```python
from build123d import *

# Parameters (mm, degrees)
F0_W      = 25
F0_H      = 60
F1_DEPTH  = 20
F2_W      = 10
F2_H      = 18
F3_DEPTH  = 25.001
F4_W      = 5
F4_H      = 7
F5_DEPTH  = 25.001
F7_D      = 3.1
F9_D      = 9.5
F9_DEPTH  = 35
F9_TIP    = 2.8540879404
F11_DEPTH = 20.001
F13_D     = 5
F13_DEPTH = 15
F13_TIP   = 1.5021515476
F14_DEPTH = 3
F15_W     = 10
F15_H     = 11
F16_DEPTH = 5.001


with BuildPart() as f1:
    # F0 (on Front) → F1 (new body)
    with BuildSketch(Plane.XZ):
        with Locations((12.5, -30)):
            Rectangle(F0_W, F0_H)
    extrude(amount=F1_DEPTH)

    # F2 (on face) → F3 (cut, through all)
    with BuildSketch(Plane(origin=(0, 0, 0), x_dir=(0, -1, 0), z_dir=(-1, 0, 0))):
        with Locations((10, -9)):
            Rectangle(F2_W, F2_H)
    extrude(amount=-F3_DEPTH, mode=Mode.SUBTRACT)

    # F4 (on face) → F5 (cut, through all)
    with BuildSketch(Plane(origin=(0, 0, 0), x_dir=(0, -1, 0), z_dir=(-1, 0, 0))):
        with Locations((2.5, -3.5)):
            Rectangle(F4_W, F4_H)
    extrude(amount=-F5_DEPTH, mode=Mode.SUBTRACT)

    # F7 (through all)
    with Locations(Plane(origin=(0, 0, 0), x_dir=(-1, 0, 0), z_dir=(0, 1, 0))):
        with Locations((-17.5, -11)):
            Hole(F7_D / 2)

    # F9
    with Locations(Plane.XY.offset(-18)):
        with Locations((5.5, -10)):
            Hole(F9_D / 2, depth=F9_DEPTH)
            with Locations((0, 0, -(F9_DEPTH + F9_TIP / 2))):  # 118° drill point
                Cone(0, F9_D / 2, F9_TIP, mode=Mode.SUBTRACT)

    # F10 (on face) → F11 (cut, through all)
    with BuildSketch(Plane.XZ.offset(20)):
        with BuildLine():
            Line((17.5, -1), (15, -1))
            ThreePointArc((15, -1), (13, -3), (15, -5))
            Line((15, -5), (17.5, -5))
            ThreePointArc((17.5, -5), (19.5, -3), (17.5, -1))
        make_face()
    extrude(amount=-F11_DEPTH, mode=Mode.SUBTRACT)

    # F13
    with Locations(Plane(origin=(0, 0, 0), x_dir=(-1, 0, 0), z_dir=(0, 1, 0))):
        with Locations((-17.5, -54), (-17.5, -22)):
            Hole(F13_D / 2, depth=F13_DEPTH)
            with Locations((0, 0, -(F13_DEPTH + F13_TIP / 2))):  # 118° drill point
                Cone(0, F13_D / 2, F13_TIP, mode=Mode.SUBTRACT)

    # F14 (add): a face of the model
    f14_faces = [f1.faces().sort_by_distance(p)[0] for p in [
        (12.5, -17.5, 0),
    ]]
    extrude(f14_faces, amount=F14_DEPTH)

    # F15 (on face) → F16 (cut, through all)
    with BuildSketch(Plane.XZ.offset(5)):
        with Locations((5, -12.5)):
            Rectangle(F15_W, F15_H)
    extrude(amount=-F16_DEPTH, mode=Mode.SUBTRACT)


solid = f1.part
```
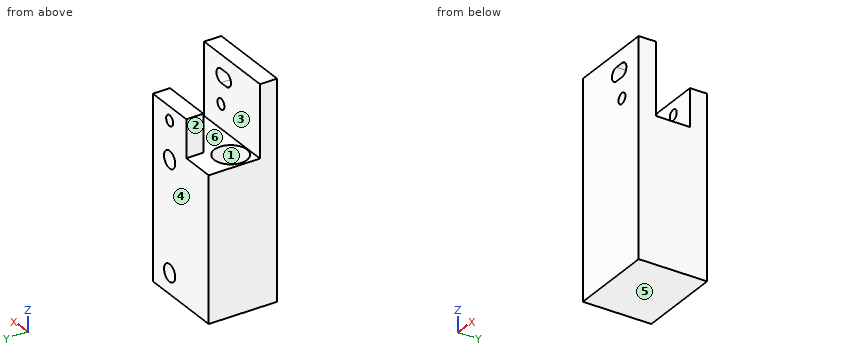
Could you check a few things on this model? Use its own coordinates, in mm. Face numbers are marked on the shaded views. A direction names the side the tool comes from. Round coordinates to 2 decimals unless told otherwise and drop trailing zeros. Order: outer loops, then holes, each group sorted by start corner. A loop starts at its lowest first (then second) coordinate and runs counter-clockwise, first axis right, second up. Notation, with made-up numbers: M 74,58 L 121,58 A24 cw 121,97 Z; hole C 40.25,65 d2. An arc over 180 degrees is marked long. One line per question, with ' | ' between items. Start each with the question number.
(1) Thinking about a two-plate mould opening in Y: for the marked faces 4, 5 and 6, which applies, +Y half, -Y half, draft (parallel to the pull), parting line (faces both ways), or undercut?
(2) Suppose I cut it at B-B on z = -37.5. List the corners of the cut face in (x, y) for me.
(3) Suppose I cut it at C-C on x = 12. List the corners of the cut face in (y, z) for me, then the cut area to 3 significant figures.
(4) Suppose I cut it at A-A on y = -4.25. List the corners of the cut face in (x, z) for me.
(5) For the marked faces 1, 2 and 3, which set-ups out of +Z, -Z, +X, -X, +Y, -Y let a thin tool reach every point of the face, with its end or its side?
(6) Suppose I cut it at D-D on z = -6. List the corners of the cut face in (x, y) for me.
(7) Please list where these lines run through material, in increasing order: line 1 along Z through (x, y) = (17.5, -9.25); line 2 along Z through (x, y) = (17.5, -17); line 3 along Z through (x, y) = (17.5, -1.45).
(8) For P1, Ø2.5, axis at y = -2.5, z = -14, coming from the -X side; P2, Ø3, axis at x = 17.5, z = -54, coming from the +Y side; P3, Ø10, axis at x = 13.5, y = -3, coming from the +Z side; P4, Ø5, axis at x = 6, z = -42.5, coming from the +Y side, each with a flat end and sliding along its axis, tell me the tip position at first contact or that it passes through.
Geometry results:
1) face 4: +Y half | face 5: draft | face 6: undercut
2) outline: M 0,-20 L 25,-20 L 25,0 L 0,0 Z; hole C 5.5,-10 d9.5
3) outline: M -20,-60 L 0,-60 L 0,-7 L -5,-7 L -5,-18 L -15,-18 L -15,3 L -20,3 Z | area: 1,000 mm²
4) outline: M 0,-60 L 25,-60 L 25,-7 L 10,-7 L 10,-18 L 0,-18 Z; hole C 17.5,-54 d5; hole C 17.5,-22 d5; hole C 17.5,-11 d3.1
5) face 1: +Z | face 2: +Z, -X, +Y | face 3: +Z, +X, -X
6) outline: M 0,-20 L 25,-20 L 25,-15 L 0,-15 Z
7) line 1: -60 to -56.5, -51.5 to -24.5, -19.5 to -18 | line 2: -60 to -12.55, -9.45 to -5, -1 to 3 | line 3: -60 to -56.5, -51.5 to -24.5, -19.5 to -12.55, -9.45 to -7
8) P1: x = 10 | P2: y = -15.6 | P3: z = -7 | P4: y = 0
